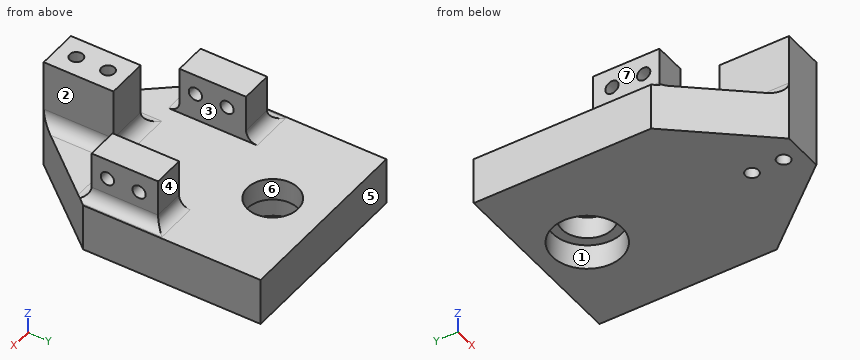
```python
from build123d import *

# Parameters (mm, degrees)
SKETCH1_W           = 60
SKETCH1_H           = 56
SKETCH1_R           = 8
BOSS_EXTRUDE1_DEPTH = 7
SKETCH2_W           = 60
SKETCH2_H           = 56
SKETCH2_R           = 11
BOSS_EXTRUDE2_DEPTH = 8
SKETCH3_W           = 10
SKETCH3_H           = 21
BOSS_EXTRUDE3_DEPTH = 15
SKETCH4_R           = 2.1
CUT_EXTRUDE1_DEPTH  = 73.249567473
SKETCH5_R           = 2.1
BOSS_EXTRUDE4_DEPTH = 15
FILLET2_R           = 3.5
BOSS_EXTRUDE5_START = 20
SKETCH7_W           = 13
SKETCH7_H           = 22
SKETCH7_R           = 2.1
BOSS_EXTRUDE5_DEPTH = 20
FILLET3_R           = 4


with BuildPart() as part:
    # Sketch1 → Boss-Extrude1 (new body)
    with BuildSketch(Plane.XY):
        with Locations((0, -12)):
            Rectangle(SKETCH1_W, SKETCH1_H)
        Circle(SKETCH1_R, mode=Mode.SUBTRACT)
    extrude(amount=BOSS_EXTRUDE1_DEPTH)

    # Sketch2 → Boss-Extrude2 (add)
    with BuildSketch(Plane(origin=(0, 0, 0), x_dir=(-1, 0, 0), z_dir=(0, 0, -1))):
        with Locations((0, -12)):
            Rectangle(SKETCH2_W, SKETCH2_H)
        Circle(SKETCH2_R, mode=Mode.SUBTRACT)
    extrude(amount=BOSS_EXTRUDE2_DEPTH)

    # Sketch3 → Boss-Extrude3 (add)
    with BuildSketch(Plane.XY.offset(7)):
        with Locations((-21, -29.5)):
            Rectangle(SKETCH3_W, SKETCH3_H)
        with Locations((21, -29.5)):
            Rectangle(SKETCH3_W, SKETCH3_H)
    extrude(amount=BOSS_EXTRUDE3_DEPTH)

    # Sketch4 → Cut-Extrude1 (cut, through all)
    with BuildSketch(Plane.ZY.offset(26)):
        with Locations((15.65, -25)):
            Circle(SKETCH4_R)
        with Locations((15.65, -35)):
            Circle(SKETCH4_R)
    extrude(amount=-CUT_EXTRUDE1_DEPTH, mode=Mode.SUBTRACT)

    # Sketch5 → Boss-Extrude4 (add, through all)
    with BuildSketch(Plane.XY.offset(7)):
        Polygon((-30, -40), (30, -40), (6.5, -68), (-6.5, -68), align=None)
        with Locations((0, -52)):
            Circle(SKETCH5_R, mode=Mode.SUBTRACT)
        with Locations((0, -62)):
            Circle(SKETCH5_R, mode=Mode.SUBTRACT)
    extrude(amount=-BOSS_EXTRUDE4_DEPTH)

    # Fillet2
    # the kernel refuses this fillet: 3.5 mm, written as the material it adds along each edge
    with BuildSketch(Plane(origin=(-26, -19, 7), x_dir=(0, 1, 0), z_dir=(1, 0, 0)), Plane(origin=(-26, -40, 7), x_dir=(0, 0, 1), z_dir=(1, 0, 0))) as fillet2_piece_1:
        with BuildLine():
            CenterArc((FILLET2_R, FILLET2_R), FILLET2_R, 180, 90)
            Line((0, FILLET2_R), (0, 0))
            Line((0, 0), (FILLET2_R, 0))
        make_face()
    extrude(amount=10)
    with BuildSketch(Plane(origin=(-26, -40, 7), x_dir=(-1, 0, 0), z_dir=(0, 1, 0))) as fillet2_piece_2:
        with BuildLine():
            CenterArc((FILLET2_R, FILLET2_R), FILLET2_R, 180, 90)
            Line((0, FILLET2_R), (0, 0))
            Line((0, 0), (FILLET2_R, 0))
        make_face()
    extrude(amount=21)
    with BuildSketch(Plane(origin=(26, -19, 7), x_dir=(0, 1, 0), z_dir=(-1, 0, 0)), Plane(origin=(16, -40, 7), x_dir=(0, -1, 0), z_dir=(1, 0, 0))) as fillet2_piece_3:
        with BuildLine():
            CenterArc((FILLET2_R, -FILLET2_R), FILLET2_R, 90, 90)
            Line((0, -FILLET2_R), (0, 0))
            Line((0, 0), (FILLET2_R, 0))
        make_face()
    extrude(amount=10)
    with BuildSketch(Plane(origin=(26, -40, 7), x_dir=(1, 0, 0), z_dir=(0, 1, 0))) as fillet2_piece_4:
        with BuildLine():
            CenterArc((FILLET2_R, -FILLET2_R), FILLET2_R, 90, 90)
            Line((0, -FILLET2_R), (0, 0))
            Line((0, 0), (FILLET2_R, 0))
        make_face()
    extrude(amount=21)
    with BuildSketch(Plane(origin=(-34.75, -19, 7), x_dir=(0, 1, 0), z_dir=(1, 0, 0))) as fillet2_piece_5a_section:
        with BuildLine():
            CenterArc((FILLET2_R, FILLET2_R), FILLET2_R, 180, 90)
            Line((0, FILLET2_R), (0, 0))
            Line((0, 0), (FILLET2_R, 0))
        make_face()
    fillet2_piece_5a = extrude(amount=18.75, mode=Mode.PRIVATE)
    fillet2_piece_5a = split(fillet2_piece_5a, bisect_by=Plane(origin=(-30, -18.2076171, 7.7923829), z_dir=(1, 0, 0)), keep=Keep.TOP, mode=Mode.PRIVATE)
    fillet2_piece_5a = split(fillet2_piece_5a, bisect_by=Plane(origin=(-26, -18.2076171, 7.7923829), z_dir=(-1, 0, 0)), keep=Keep.TOP, mode=Mode.PRIVATE)
    with BuildSketch(Plane(origin=(-26, -40, 7), x_dir=(-1, 0, 0), z_dir=(0, 1, 0))) as fillet2_piece_5b_section:
        with BuildLine():
            CenterArc((FILLET2_R, FILLET2_R), FILLET2_R, 180, 90)
            Line((0, FILLET2_R), (0, 0))
            Line((0, 0), (FILLET2_R, 0))
        make_face()
    fillet2_piece_5b = extrude(amount=29.75, mode=Mode.PRIVATE)
    fillet2_piece_5b = split(fillet2_piece_5b, bisect_by=Plane(origin=(-26.7923829, -19, 7.7923829), z_dir=(0, 1, 0)), keep=Keep.TOP, mode=Mode.PRIVATE)
    fillet2_piece_5 = fillet2_piece_5a & fillet2_piece_5b
    add(fillet2_piece_5)
    with BuildSketch(Plane(origin=(-34.75, -40, 7), x_dir=(0, 0, 1), z_dir=(1, 0, 0))) as fillet2_piece_6a_section:
        with BuildLine():
            CenterArc((FILLET2_R, FILLET2_R), FILLET2_R, 180, 90)
            Line((0, FILLET2_R), (0, 0))
            Line((0, 0), (FILLET2_R, 0))
        make_face()
    fillet2_piece_6a = extrude(amount=18.75, mode=Mode.PRIVATE)
    fillet2_piece_6a = split(fillet2_piece_6a, bisect_by=Plane(origin=(-26, -40.649592252, 7.87643738), z_dir=(-1, 0, 0)), keep=Keep.TOP, mode=Mode.PRIVATE)
    fillet2_piece_6a = split(fillet2_piece_6a, bisect_by=Plane(origin=(-28.740316489, -41.500899502, 7.87643738), z_dir=(0.765974253829985, 0.6428712487501661, 0)), keep=Keep.TOP, mode=Mode.PRIVATE)
    fillet2_piece_6a = split(fillet2_piece_6a, bisect_by=Plane(origin=(-30, -40.649592252, 7.87643738), z_dir=(1, 0, 0)), keep=Keep.TOP, mode=Mode.PRIVATE)
    with BuildSketch(Plane(origin=(-26, -48.75, 7), x_dir=(-1, 0, 0), z_dir=(0, 1, 0))) as fillet2_piece_6b_section:
        with BuildLine():
            CenterArc((FILLET2_R, FILLET2_R), FILLET2_R, 180, 90)
            Line((0, FILLET2_R), (0, 0))
            Line((0, 0), (FILLET2_R, 0))
        make_face()
    fillet2_piece_6b = extrude(amount=29.75, mode=Mode.PRIVATE)
    fillet2_piece_6b = split(fillet2_piece_6b, bisect_by=Plane(origin=(-26.614887028, -40, 7.897241021), z_dir=(0, -1, 0)), keep=Keep.TOP, mode=Mode.PRIVATE)
    fillet2_piece_6b = split(fillet2_piece_6b, bisect_by=Plane(origin=(-27.607937943, -42.850116494, 7.897241021), z_dir=(0.765974253829985, 0.6428712487501661, 0)), keep=Keep.TOP, mode=Mode.PRIVATE)
    fillet2_piece_6 = fillet2_piece_6a & fillet2_piece_6b
    add(fillet2_piece_6)
    with BuildSketch(Plane(origin=(26, -40, 7), x_dir=(1, 0, 0), z_dir=(0, 1, 0))) as fillet2_piece_7a_section:
        with BuildLine():
            CenterArc((FILLET2_R, -FILLET2_R), FILLET2_R, 90, 90)
            Line((0, -FILLET2_R), (0, 0))
            Line((0, 0), (FILLET2_R, 0))
        make_face()
    fillet2_piece_7a = extrude(amount=29.75, mode=Mode.PRIVATE)
    fillet2_piece_7a = split(fillet2_piece_7a, bisect_by=Plane(origin=(26.7923829, -19, 7.7923829), z_dir=(0, 1, 0)), keep=Keep.TOP, mode=Mode.PRIVATE)
    with BuildSketch(Plane(origin=(34.75, -19, 7), x_dir=(0, 1, 0), z_dir=(-1, 0, 0))) as fillet2_piece_7b_section:
        with BuildLine():
            CenterArc((FILLET2_R, -FILLET2_R), FILLET2_R, 90, 90)
            Line((0, -FILLET2_R), (0, 0))
            Line((0, 0), (FILLET2_R, 0))
        make_face()
    fillet2_piece_7b = extrude(amount=18.75, mode=Mode.PRIVATE)
    fillet2_piece_7b = split(fillet2_piece_7b, bisect_by=Plane(origin=(30, -18.2076171, 7.7923829), z_dir=(-1, 0, 0)), keep=Keep.TOP, mode=Mode.PRIVATE)
    fillet2_piece_7b = split(fillet2_piece_7b, bisect_by=Plane(origin=(26, -18.2076171, 7.7923829), z_dir=(1, 0, 0)), keep=Keep.TOP, mode=Mode.PRIVATE)
    fillet2_piece_7 = fillet2_piece_7a & fillet2_piece_7b
    add(fillet2_piece_7)
    with BuildSketch(Plane(origin=(16, -40, 7), x_dir=(0, -1, 0), z_dir=(1, 0, 0))) as fillet2_piece_8a_section:
        with BuildLine():
            CenterArc((FILLET2_R, -FILLET2_R), FILLET2_R, 90, 90)
            Line((0, -FILLET2_R), (0, 0))
            Line((0, 0), (FILLET2_R, 0))
        make_face()
    fillet2_piece_8a = extrude(amount=18.75, mode=Mode.PRIVATE)
    fillet2_piece_8a = split(fillet2_piece_8a, bisect_by=Plane(origin=(28.740316489, -41.500899502, 7.87643738), z_dir=(-0.7659742538299851, 0.6428712487501659, 0)), keep=Keep.TOP, mode=Mode.PRIVATE)
    fillet2_piece_8a = split(fillet2_piece_8a, bisect_by=Plane(origin=(30, -40.649592252, 7.87643738), z_dir=(-1, 0, 0)), keep=Keep.TOP, mode=Mode.PRIVATE)
    fillet2_piece_8a = split(fillet2_piece_8a, bisect_by=Plane(origin=(26, -40.649592252, 7.87643738), z_dir=(1, 0, 0)), keep=Keep.TOP, mode=Mode.PRIVATE)
    with BuildSketch(Plane(origin=(26, -48.75, 7), x_dir=(1, 0, 0), z_dir=(0, 1, 0))) as fillet2_piece_8b_section:
        with BuildLine():
            CenterArc((FILLET2_R, -FILLET2_R), FILLET2_R, 90, 90)
            Line((0, -FILLET2_R), (0, 0))
            Line((0, 0), (FILLET2_R, 0))
        make_face()
    fillet2_piece_8b = extrude(amount=29.75, mode=Mode.PRIVATE)
    fillet2_piece_8b = split(fillet2_piece_8b, bisect_by=Plane(origin=(27.607937943, -42.850116494, 7.897241021), z_dir=(-0.7659742538299851, 0.6428712487501659, 0)), keep=Keep.TOP, mode=Mode.PRIVATE)
    fillet2_piece_8b = split(fillet2_piece_8b, bisect_by=Plane(origin=(26.614887028, -40, 7.897241021), z_dir=(0, -1, 0)), keep=Keep.TOP, mode=Mode.PRIVATE)
    fillet2_piece_8 = fillet2_piece_8a & fillet2_piece_8b
    add(fillet2_piece_8)

    # Sketch7 → Boss-Extrude5 (add)
    with BuildSketch(Plane.XY.offset(7).offset(BOSS_EXTRUDE5_START)):
        with Locations((0, -57)):
            Rectangle(SKETCH7_W, SKETCH7_H)
        with Locations((0, -62)):
            Circle(SKETCH7_R, mode=Mode.SUBTRACT)
        with Locations((0, -52)):
            Circle(SKETCH7_R, mode=Mode.SUBTRACT)
    extrude(amount=-BOSS_EXTRUDE5_DEPTH)

    # Fillet3
    fillet3_edges = [part.edges().sort_by_distance(p)[0] for p in [
        (-6.5, -57, 7),
        (6.5, -57, 7),
        (0, -46, 7),
    ]]
    fillet(fillet3_edges, radius=FILLET3_R)


solid = part.part
```
Read the model definition and answer for the solid it produces. Units are mm, in the model's axes. Face numbers are marked on the shaded views. A direction names the side the tool comes from. Round coordinates to 2 decimals unless told otherwise and drop trailing zeros. Write each loop counter-clockwise with the first axis right and the second up, starting at its lowest first coordinate (ties: lowest second). Pieces come first, ordered by that corner, then holes. Notation, with made-up numbers: (47, 49.5) -> (62, 49.5) arc R19 ccw to (62, 69.5) -> close; hole circle Ø2 at (-33, -0.5). An arc over 180 degrees is marked (long way). Answer in a Markdown table with one row per item. Add a question column.
1) Find section A-A, the plane x = 0. Determine the outline of the cut face in (y, z), and give its area (3 significant figures).
2) Which of the six approach directions +Z, -Z, +X, -X, +Y, -Y give full straight-line access (tool end or side, diameter ignored) to the marked faces 1, 2, 3 and 4?
3) Consider line 1 (Y direction, x = 20.25, z = 15.65); line 2 (Y direction, x = 0, z = 4.75); line 3 (Y direction, x = 0, z = -2.25). Determine where each line is inside the solid, lowest interval first.
4) Find section D-D, the plane y = 0. Determine the outline of the cut face in (x, z), and give its area (3 significant figures).
5) Find section B-B, the plane y = -25. Determine the outline of the cut face in (x, z), and give its area (3 significant figures).
6) Determine the mould class of the marked faces 5, 6 and 7 for opening direction Y: pulls with the +Y half, pulls with the -Y half, needs draft (parallel to the pull), parting line crosses it, or undercut.
7) Find section C-C, the plane z = 24.5. Determine the outline of the cut face in (x, y).
8) Given P1, Ø3, axis at x = -21, z = 18.5, coming from the +Y side; P2, Ø10, axis at y = -46.5, z = 10, coming from the +X side; P3, Ø11, axis at x = 23, z = 17.5, coming from the -Y side, each flat-ended and moving along its own axis, determine where each tip first touches the part or whether it passes through.
Findings below:
| question | item | result |
|---|---|---|
| 1 | outline | (-68, -8) -> (-64.1, -8) -> (-64.1, 27) -> (-68, 27) -> close; (-59.9, -8) -> (-54.1, -8) -> (-54.1, 27) -> (-59.9, 27) -> close; (-49.9, -8) -> (-11, -8) -> (-11, 0) -> (-8, 0) -> (-8, 7) -> (-42, 7) arc R4 cw to (-46, 11) -> (-46, 27) -> (-49.9, 27) -> close; (8, 0) -> (11, 0) -> (11, -8) -> (16, -8) -> (16, 7) -> (8, 7) -> close |
| 1 | area | 1,120 mm² |
| 2 | face 1 | -Z |
| 2 | face 2 | +Z, +X, +Y, -Y |
| 2 | face 3 | +Z, +Y, -Y |
| 2 | face 4 | +Z, +X, -X, +Y |
| 3 | line 1 | -40 to -37.1, -32.9 to -27.1, -22.9 to -19 |
| 3 | line 2 | -68 to -64.1, -59.9 to -54.1, -49.9 to -8, 8 to 16 |
| 3 | line 3 | -68 to -64.1, -59.9 to -54.1, -49.9 to -11, 11 to 16 |
| 4 | outline | (-30, -8) -> (-11, -8) -> (-11, 0) -> (-8, 0) -> (-8, 7) -> (-30, 7) -> close; (8, 0) -> (11, 0) -> (11, -8) -> (30, -8) -> (30, 7) -> (8, 7) -> close |
| 4 | area | 612 mm² |
| 5 | outline | (-30, -8) -> (30, -8) -> (30, 7) -> (29.5, 7) arc R3.5 cw to (26, 10.5) -> (26, 13.55) -> (16, 13.55) -> (16, 7) -> (-16, 7) -> (-16, 13.55) -> (-26, 13.55) -> (-26, 10.5) arc R3.5 cw to (-29.5, 7) -> (-30, 7) -> close; (-26, 17.75) -> (-16, 17.75) -> (-16, 22) -> (-26, 22) -> close; (16, 17.75) -> (26, 17.75) -> (26, 22) -> (16, 22) -> close |
| 5 | area | 1,120 mm² |
| 6 | face 5 | pulls with the +Y half |
| 6 | face 6 | undercut |
| 6 | face 7 | needs draft |
| 7 | outline | (-6.5, -68) -> (6.5, -68) -> (6.5, -46) -> (-6.5, -46) -> close; hole circle Ø4.2 at (0, -62); hole circle Ø4.2 at (0, -52) |
| 8 | P1 | y = -19 |
| 8 | P2 | x = 28.02 |
| 8 | P3 | y = -40 |
